Job drawing, mm, ordinate dimensions from the low corner. One solid piece. Coordinates: 2 decimals unless noted, no trailing zeros. Loops run counter-clockwise (first coordinate to the right, second up) from the corner with the lowest first, then second, coordinate; pieces in that order, holes last. Notation, with made-up numbers: (-12, 71.25) - (21, 71.25) arc R14 ccw to (21, 94.25) - close; hole circle Ø7 at (-11, 0). An arc over 180 degrees is marked (long way). Use a Markdown table: item, result. Add a question column.
1) Band-saw the part on B-B (z = 2.25). Give the cut face in (x, y), plus the area to 3 significant figures.
2) Pull direction X, two halves, no side cores. Call the marked faces 1, 2 and 3: +X half, -X half, draft (parallel to the pull), parting line (faces both ways), or undercut.
3) Band-saw the part on C-C (x = 8). Give the cut face in (y, z).
4) Band-saw the part on A-A (y = 0.4). Give the cut face in (x, z), plus the area to 3 significant figures.
5) Probe probe 1 along Y at (x, z) = (7.25, 2); probe 2 along Y at (x, z) = (7.5, 9). List the from-to ranges inside material, lowest first. Write a range as [from, to].
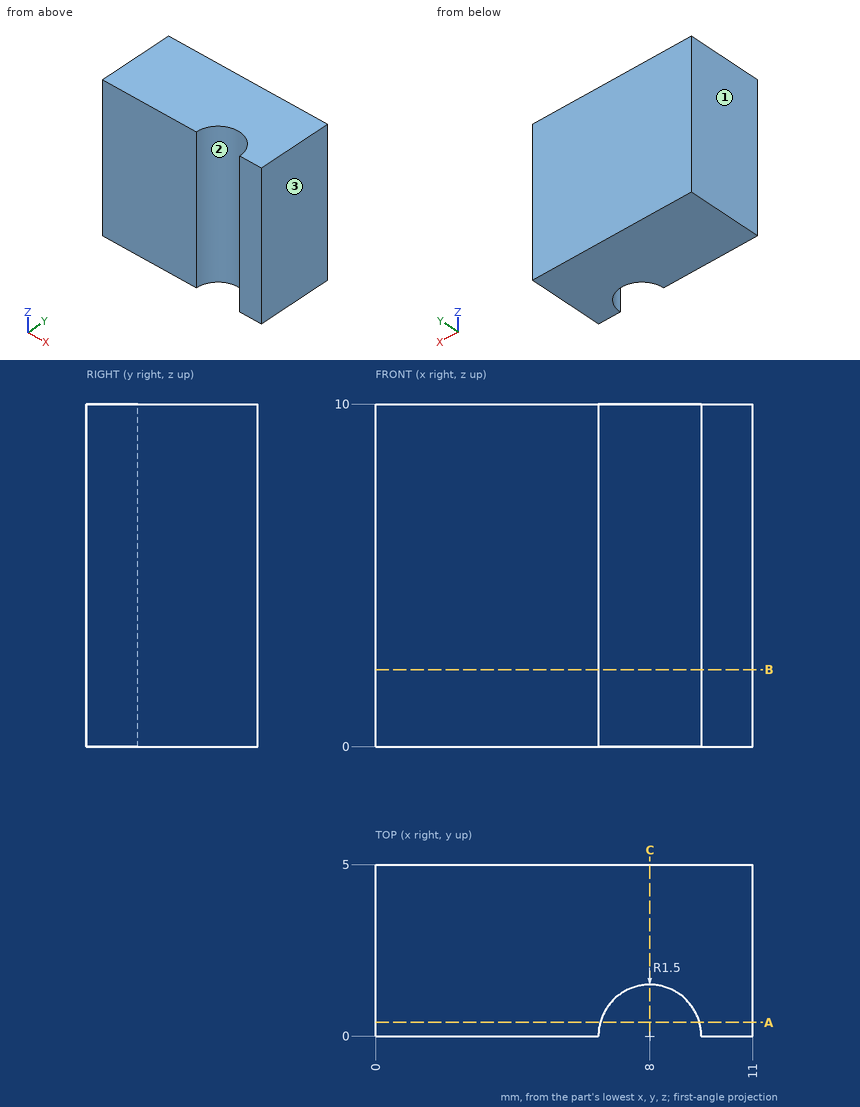
Answer block:
| question | item | result |
|---|---|---|
| 1 | outline | (0, 0) - (6.5, 0) arc R1.5 cw to (9.5, 0) - (11, 0) - (11, 5) - (0, 5) - close |
| 1 | area | 51.5 mm2 |
| 2 | face 1 | -X half |
| 2 | face 2 | undercut |
| 2 | face 3 | +X half |
| 3 | outline | (1.5, 0) - (5, 0) - (5, 10) - (1.5, 10) - close |
| 4 | outline | (0, 0) - (6.55, 0) - (6.55, 10) - (0, 10) - close; (9.45, 0) - (11, 0) - (11, 10) - (9.45, 10) - close |
| 4 | area | 81.1 mm2 |
| 5 | probe 1 | [1.3, 5] |
| 5 | probe 2 | [1.41, 5] |
